from build123d import *

# Parameters (mm, degrees)
SKETCH_1_R          = 2.8
EXTRUDE_1_DEPTH     = 3
CUT_EXTRUDE_1_DEPTH = 1.5
SKETCH_3_R          = 1.4
EXTRUDE_2_DEPTH     = 10
CHAMFER_1_SIZE      = 0.1


with BuildPart() as part:
    # 草图1 → 凸台-拉伸1 (new body)
    with BuildSketch(Plane(origin=(0, 0, 0), x_dir=(1, 0, 0), z_dir=(0, 1, 0))):
        Circle(SKETCH_1_R)
    extrude(amount=EXTRUDE_1_DEPTH)

    # 草图2 → 切除-拉伸1 (cut)
    with BuildSketch(Plane(origin=(0, 3, 0), x_dir=(1, 0, 0), z_dir=(0, 1, 0))):
        Polygon((0, -1.489563695), (1.29, -0.744781847), (1.29, 0.744781847), (0, 1.489563695), (-1.29, 0.744781847), (-1.29, -0.744781847), align=None)
    extrude(amount=-CUT_EXTRUDE_1_DEPTH, mode=Mode.SUBTRACT)

    # 草图3 → 凸台-拉伸2 (add)
    with BuildSketch(Plane.XZ):
        Circle(SKETCH_3_R)
    extrude(amount=EXTRUDE_2_DEPTH)

    # 倒角1
    chamfer_1_edges = [part.edges().sort_by_distance(p)[0] for p in [
        (-0.645, 3, 1.117172771),
        (0.645, 3, 1.117172771),
        (1.29, 3, 0),
        (0.645, 3, -1.117172771),
        (-0.645, 3, -1.117172771),
        (-1.29, 3, 0),
        (-1.4, -10, 0),
    ]]
    chamfer(chamfer_1_edges, length=CHAMFER_1_SIZE)


solid = part.part
Input: part model. Units: mm. Frame: model coordinates. A direction names the side the tool comes from. Coordinates: 2 decimals unless noted, no trailing zeros. Loops run counter-clockwise (first coordinate to the right, second up) from the corner with the lowest first, then second, coordinate; pieces in that order, holes last.
Q1. Set-up query: faces 1 (the face through (1.2, 3, 1.2)), 2 (the face through (-1.4, -4.88, 0.06)), 3 (the face through (0.64, 2.21, 1.12)). Return all of +Z, -Z, +X, -X, +Y, -Y with unobstructed straight access to the full face (end or side cutting, diameter ignored); none if empty.
Q2. Material intervals for line 1 (Y direction, x = 0.6, z = 1.35); line 2 (Y direction, x = 0.45, z = -0.4); line 3 (Z direction, x = 0.05, y = -7.5), sorted ascending.
Q3. Cut plane C-C (x = -1.65). Output: boundary loops of the cut face in (y, z), then the cut area to 3 significant figures.
Q4. Cut plane D-D (y = 1.25). Output: boundary loops of the cut face in (x, z).
Q5. Cut plane A-A (z = 0). Output: boundary loops of the cut face in (x, y), then the cut area to 3 significant figures.
Q6. Contact query for flat-ended pins moving along their axis: pin 1 (2 mm diameter, centred on x = -2, y = -0.5, fed in from -Z); pin 2 (3 mm diameter, centred on y = -7, z = -0.5, fed in from +X); pin 3 (0.7 mm diameter, centred on y = 2, z = 0.5, fed in from +X). Output: stop coordinate, or through.
Q7. Draft query along X for faces 4 (the face through (-2.8, 1.5, -0.1)), 5 (the face through (0, -10, 0)), 6 (the face through (1.29, 2, 0)). Return one class per face: +X half, -X half, draft (parallel to the pull), parting line (faces both ways), or undercut.
Q8. Cut plane B-B (y = -8). Output: boundary loops of the cut face in (x, z), then the cut area to 3 significant figures.
Working result:
1. face 1: +Z, -Z, +X, -X, +Y
1. face 2: -Y
1. face 3: +Y
2. line 1: y = 0 to 3
2. line 2: y = -10 to 1.5
2. line 3: z = -1.4 to 1.4
3. outline: (0, -2.26) - (3, -2.26) - (3, 2.26) - (0, 2.26) - close
3. area: 13.6 mm2
4. outline: circle Ø5.6 at (0, 0)
5. outline: (-2.8, 0) - (-1.4, 0) - (-1.4, -9.9) - (-1.3, -10) - (1.3, -10) - (1.4, -9.9) - (1.4, 0) - (2.8, 0) - (2.8, 3) - (1.39, 3) - (1.29, 2.9) - (1.29, 1.5) - (-1.29, 1.5) - (-1.29, 2.9) - (-1.39, 3) - (-2.8, 3) - close
5. area: 40.9 mm2
6. pin 1: stops at z = -2.56
6. pin 2: stops at x = 1.4
6. pin 3: stops at x = 2.8
7. face 4: parting line
7. face 5: draft
7. face 6: undercut
8. outline: circle Ø2.8 at (0, 0)
8. area: 6.16 mm2
